```python
from build123d import *

# Parameters (mm, degrees)
SKETCH_1_R      = 7.9
EXTRUDE_1_DEPTH = 15


with BuildPart() as part:
    # 草图1 → 凸台-拉伸1 (new body)
    with BuildSketch(Plane.XY):
        Circle(SKETCH_1_R)
        with BuildLine():
            Line((-5.082, 3.282647712), (-5.082, -3.282647712))
            ThreePointArc((-5.082, -3.282647712), (0, -6.05), (5.082, -3.282647712))
            Line((5.082, -3.282647712), (5.082, 3.282647712))
            ThreePointArc((5.082, 3.282647712), (0, 6.05), (-5.082, 3.282647712))
        make_face(mode=Mode.SUBTRACT)
    extrude(amount=EXTRUDE_1_DEPTH)


solid = part.part
```
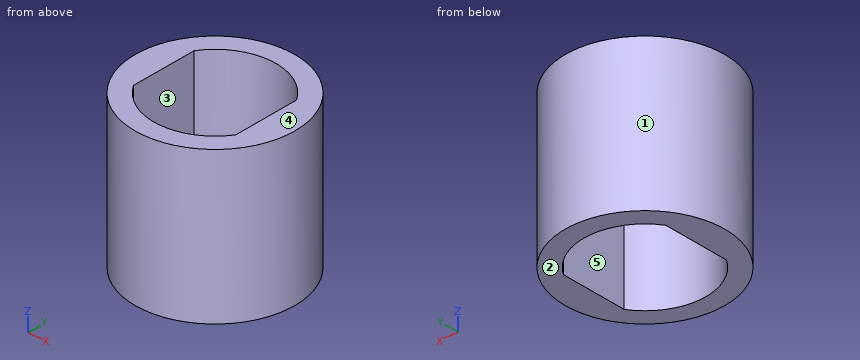
Build history of the part. All positions in model axes, mm. Face numbers are marked on the shaded views. A direction names the side the tool comes from. Round coordinates to 2 decimals unless told otherwise and drop trailing zeros. Loops run counter-clockwise (first coordinate to the right, second up) from the corner with the lowest first, then second, coordinate; pieces in that order, holes last. Notation, with made-up numbers: M -37,79 L 17,79 A17 cw 17,107 Z; hole C -39.75,71.5 d9. An arc over 180 degrees is marked long. Answer as CSV lines item,"result".
1. Two-plate mould, pull along X, no slides. Class the marked faces 1, 2 and 3: released by +X, released by -X, zero draft, split by the parting line, or undercut.
Resolved:
face 1,"split by the parting line"
face 2,"zero draft"
face 3,"undercut"
2. Cut at C-C on z = 1. Write the cut outline in (x, y).
Resolved:
outline,"C 0,0 d15.8; hole M -5.08,-3.28 A6.05 ccw 5.08,-3.28 L 5.08,3.28 A6.05 ccw -5.08,3.28 Z"
3. 3-axis set-ups, long thin cutter, end or side, ignore diameter. For the marked faces 4 and 5: which of +Z, -Z, +X, -X, +Y, -Y reach the whole face in a straight line?
Resolved:
face 4,"+Z, +X, -X, +Y, -Y"
face 5,"+Z, -Z"
4. Flat gauge pins, fed straight in: P1, Ø1, axis at x = 3, z = 11.5, coming from the -Y side; P2, Ø1.5, axis at y = 4, z = 11.5, coming from the +X side; P3, Ø5.5, axis at y = -1.5, z = 8.5, coming from the -X side; P4, Ø6, axis at y = 4.5, z = 3, coming from the +X side. Where does each tip first touch, or does it go through?
Resolved:
P1,"stops at y = -7.49"
P2,"stops at x = 7.2"
P3,"stops at x = -7.9"
P4,"stops at x = 7.76"
5. Wall check: probe 1 along Y at (x, z) = (3, 8.75); probe 2 along X at (y, z) = (1.25, 2.25); probe 3 along X at (y, z) = (5.25, 7.5). Give the ranges that are in metal, low to high. Write a range as [from, to].
Resolved:
probe 1,"y = [-7.31, -5.25], [5.25, 7.31]"
probe 2,"x = [-7.8, -5.08], [5.08, 7.8]"
probe 3,"x = [-5.9, -3.01], [3.01, 5.9]"
6. Cut at D-D on x = 6.5. Write the cut outline in (y, z).
Resolved:
outline,"M -4.49,0 L 4.49,0 L 4.49,15 L -4.49,15 Z"
7. Cut at B-B on y = 0. Write the cut outline in (x, z).
Resolved:
outline,"M -7.9,0 L -5.08,0 L -5.08,15 L -7.9,15 Z; M 5.08,0 L 7.9,0 L 7.9,15 L 5.08,15 Z"
8. Cut at A-A on x = 0. Write the cut outline in (y, z), then the cut area to 3 significant figures.
Resolved:
outline,"M -7.9,0 L -6.05,0 L -6.05,15 L -7.9,15 Z; M 6.05,0 L 7.9,0 L 7.9,15 L 6.05,15 Z"
area,"55.5 mm²"
